Geometry check sheet. Reference: the model listing, model coordinates, mm. Give positions to 0.01 mm unless a question says otherwise; leave off trailing zeros. Loops run counter-clockwise (first coordinate to the right, second up) from the corner with the lowest first, then second, coordinate; pieces in that order, holes last. Notation, with made-up numbers: (67, 60.5) -> (87, 60.5) arc R6 cw to (87, 69.5) -> close; hole circle Ø4 at (16, -8). An arc over 180 degrees is marked (long way). One line per question, with ' | ' between items.
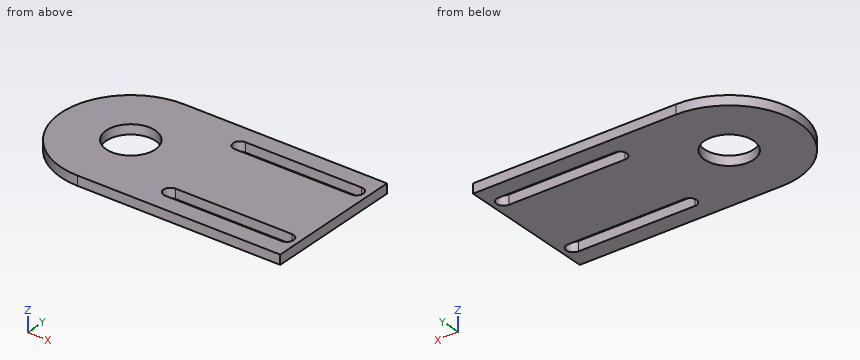
Autodesk Inventor part; units mm, degrees
ref_plane "YZ Plane" through (0, 0, 0) normal (1, 0, 0) x (0, 1, 0)
ref_plane "XZ Plane" through (0, 0, 0) normal (0, 1, 0) x (-1, 0, 0)
ref_plane "XY Plane" through (0, 0, 0) normal (0, 0, 1) x (1, 0, 0)
ref_plane "Work Plane1" through (0, 0, 0) normal (0, 0, 1) x (1, 0, 0)
sketch "Sketch1" plane through (0, 0, 0) normal (0, 0, 1) x (1, 0, 0)
  line L0 (11.43, 0) -> (11.43, -63.5) construction
  line L1 (0, 0) -> (11.43, 0) construction
  line L2 (0, 0) -> (0, -63.5) construction
  line L3 (7.44, -34.7378) -> (0, -34.7378) construction
  circle A0 centre (5.715, -31.75) radius 1.7 construction
  circle A1 centre (-31.5722, -43.7048) radius 6.4135
  line L4 (0, -63.5) -> (11.43, -63.5) construction
  circle A2 centre (5.715, -55.6597) radius 1.7 construction
  line L5 (21.59, -62.0097) -> (-31.5722, -62.0097)
  line L6 (-31.5722, -25.4) -> (21.59, -25.4)
  line L7 (21.59, -25.4) -> (21.59, -62.0097)
  arc A3 (-31.5722, -25.4) -> (-31.5722, -62.0097) centre (-31.5722, -43.7048) ccw
  line L8 (18.415, -31.75) -> (-12.065, -31.75) construction
  line L9 (18.415, -29.95) -> (-12.065, -29.95)
  line L10 (-12.065, -33.55) -> (18.415, -33.55)
  arc A4 (18.415, -33.55) -> (18.415, -29.95) centre (18.415, -31.75) ccw
  arc A5 (-12.065, -29.95) -> (-12.065, -33.55) centre (-12.065, -31.75) ccw
  line L11 (18.415, -55.6597) -> (-12.065, -55.6597) construction
  line L12 (18.415, -53.8597) -> (-12.065, -53.8597)
  line L13 (-12.065, -57.4597) -> (18.415, -57.4597)
  arc A6 (18.415, -57.4597) -> (18.415, -53.8597) centre (18.415, -55.6597) ccw
  arc A7 (-12.065, -53.8597) -> (-12.065, -57.4597) centre (-12.065, -55.6597) ccw
  point P0 (3.175, -31.75)
  point P1 (3.175, -55.6597)
extrude "Extrusion1" add sketch "Sketch1" along normal blind 2.5
equation "\"d3\" = d4 + 0.5 * d5"
properties part number "driven wheel arm"
Item 1: Scan lines: probe 1 along Y at (x, z) = (0, 1.9); probe 2 along X at (y, z) = (-40, 0.3); probe 3 along X at (y, z) = (-32.5, 0.7). Record each from-to range of solid material in increasing order.
Result:
probe 1: -62.01 to -57.46, -53.86 to -33.55, -29.95 to -25.4 | probe 2: -49.5 to -36.81, -26.34 to 21.59 | probe 3: -46.05 to -13.7, 20.05 to 21.59
Item 2: Sectioned sample at B-B (y = -38). Record the cut outline in (x, z), plus the area to 3 significant figures.
Result:
outline: (-48.97, 0) -> (-34.5, 0) -> (-34.5, 2.5) -> (-48.97, 2.5) -> close; (-28.64, 0) -> (21.59, 0) -> (21.59, 2.5) -> (-28.64, 2.5) -> close | area: 162 mm2
Item 3: Depth check by flat-ended pin: pin 1 Ø1 at (y, z) = (-39.5, 1.5) entering from -X; pin 2 Ø10.5 at (x, y) = (-31.57, -43.7) entering from -Z. Enter the tip coordinate at first touch or a pass-through.
Result:
pin 1: x = -49.5 | pin 2: through
Item 4: Sectioned sample at A-A (x = -2.5). Record the cut outline in (y, z), plus the area to 3 significant figures.
Result:
outline: (-62.01, 0) -> (-57.46, 0) -> (-57.46, 2.5) -> (-62.01, 2.5) -> close; (-53.86, 0) -> (-33.55, 0) -> (-33.55, 2.5) -> (-53.86, 2.5) -> close; (-29.95, 0) -> (-25.4, 0) -> (-25.4, 2.5) -> (-29.95, 2.5) -> close | area: 73.5 mm2
Item 5: Sectioned sample at D-D (y = -31.75). Record the cut outline in (x, z) (3 decimals), plus the area to 3 significant figures.
Result:
outline: (-45.434, 0) -> (-13.865, 0) -> (-13.865, 2.5) -> (-45.434, 2.5) -> close; (20.215, 0) -> (21.59, 0) -> (21.59, 2.5) -> (20.215, 2.5) -> close | area: 82.4 mm2
Item 6: Sectioned sample at C-C (z = 0.65). Give the number of separate pieces and of enclosed holes in the cut face, plus the area to 3 significant figures.
Result:
separate pieces: 1 | enclosed holes: 3 | area: 2,100 mm2
